```python
from build123d import *

# Parameters (mm, degrees)
HEAD_DEPTH         = 5.2
HOLE_SKETCH_R      = 3
THROUGH_HOLE_DEPTH = 6.2000001


with BuildPart() as part:
    # Head Sketch → Head (new body)
    with BuildSketch(Plane.XY):
        Polygon((0, 5.773502692), (5, 2.886751346), (5, -2.886751346), (0, -5.773502692), (-5, -2.886751346), (-5, 2.886751346), align=None)
    extrude(amount=HEAD_DEPTH)

    # Sketch5 → Head Trim (revolve, cut)
    with BuildSketch(Plane(origin=(0, 0, 0), x_dir=(0, 0, -1), z_dir=(1, 0, 0))):
        with BuildLine():
            Line((-5.2, -4.773502692), (-5.2, -5.773502692))
            Line((-5.2, -5.773502692), (-4.2, -5.773502692))
            ThreePointArc((-4.2, -5.773502692), (-4.907106781, -5.480609473), (-5.2, -4.773502692))
        make_face()
    head_trim = revolve(axis=Axis((0, 0, 15.085599173), (0, 0, -1)), mode=Mode.SUBTRACT)

    # Hole Sketch → Through Hole (cut, through all)
    with BuildSketch(Plane.XY.offset(5.2)):
        Circle(HOLE_SKETCH_R)
    extrude(amount=-THROUGH_HOLE_DEPTH, mode=Mode.SUBTRACT)

    # Symétrie2: Head Trim across plane
    add(head_trim.mirror(Plane.XY.offset(2.6)), mode=Mode.SUBTRACT)


solid = part.part
```
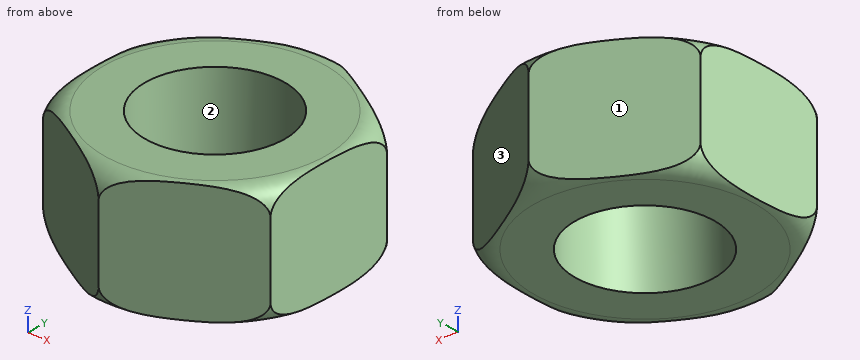
Geometry: final body of the model. Coordinates: model frame, mm. Face numbers are marked on the shaded views. Round coordinates to 2 decimals unless told otherwise and drop trailing zeros. Loops run counter-clockwise (first coordinate to the right, second up) from the corner with the lowest first, then second, coordinate; pieces in that order, holes last. Notation, with made-up numbers: (42.5, 44.25) -> (89.5, 44.25) arc R15 cw to (89.5, 70.25) -> close; hole circle Ø1 at (-6.75, -2.75). An arc over 180 degrees is marked (long way). Use one line per item in the form item = value. Start each with the question number.
1) First-contact query: P1, Ø3, axis at x = -0.5, y = 2.5, coming from the +Z side. Flat tip, straight axial feed; report the tip coordinate or a pass-through.
2) Section B-B on z = 3.6. Output: boundary loops of the cut face in (x, y).
3) Section A-A on y = 0. Output: boundary loops of the cut face in (x, z), then the cut area to 3 significant figures.
4) Draft query along X for the marked faces 1, 2 and 3. Return one class per face: released by +X, released by -X, zero draft, split by the parting line, or undercut.
5) Line query: L1, parallel to X at y = -1.25, z = 4.95; L2, parallel to Y at x = -1.75, z = 2.9; L3, parallel to X at y = 2.5, z = 2.05. Output: solid intervals per line, ascending.
6) Section C-C on z = 4.7. Output: boundary loops of the cut face in (x, y).
Response:
q1.P1 = 5.2
q2.outline = (-5, -2.89) -> (0, -5.77) -> (5, -2.89) -> (5, 2.89) -> (0, 5.77) -> (-5, 2.89) -> close; hole circle Ø6 at (0, 0)
q3.outline = (-5, 0.03) arc R1 ccw to (-4.77, 0) -> (-3, 0) -> (-3, 5.2) -> (-4.77, 5.2) arc R1 ccw to (-5, 5.17) -> close; (3, 0) -> (4.77, 0) arc R1 ccw to (5, 0.03) -> (5, 5.17) arc R1 ccw to (4.77, 5.2) -> (3, 5.2) -> close
q3.area = 20.8 mm^2
q4.face_1 = released by -X
q4.face_2 = undercut
q4.face_3 = released by +X
q5.L1 = -5 to -2.73, 2.73 to 5
q5.L2 = -4.76 to -2.44, 2.44 to 4.76
q5.L3 = -5 to -1.66, 1.66 to 5
q6.outline = (-5, -2.61) arc R5.64 ccw to (-4.76, -3.03) -> (-0.24, -5.63) arc R5.64 ccw to (0.24, -5.63) -> (4.76, -3.03) arc R5.64 ccw to (5, -2.61) -> (5, 2.61) arc R5.64 ccw to (4.76, 3.03) -> (0.24, 5.63) arc R5.64 ccw to (-0.24, 5.63) -> (-4.76, 3.03) arc R5.64 ccw to (-5, 2.61) -> close; hole circle Ø6 at (0, 0)
